Part model, mm, in its own coordinate system. Face numbers are marked on the shaded views. A direction names the side the tool comes from. Give positions to 0.01 mm unless a question says otherwise; leave off trailing zeros. Order: outer loops, then holes, each group sorted by start corner. A loop starts at its lowest first (then second) coordinate and runs counter-clockwise, first axis right, second up. Notation, with made-up numbers: (1.5, -8.5) - (31.5, -8.5) arc R17 cw to (31.5, 20.5) - close; hole circle Ø4 at (50, 31). An arc over 180 degrees is marked (long way). One line per item, written item: value.
```python
from build123d import *

# Parameters (mm, degrees)
SKETCH1_R           = 25
SKETCH1_R_2         = 22.5
BOSS_EXTRUDE1_DEPTH = 9.4
SKETCH2_R           = 25
BOSS_EXTRUDE2_DEPTH = 40
SKETCH3_W           = 55.38055132
SKETCH3_H           = 33.998264421
CUT_EXTRUDE1_DEPTH  = 36
SKETCH4_R           = 3.5
CUT_EXTRUDE2_DEPTH  = 36
CUT_EXTRUDE3_START  = -2
SKETCH5_R           = 3.5
SKETCH5_R_2         = 2.05
SKETCH5_R_3         = 1.95
CUT_EXTRUDE3_DEPTH  = 2
SKETCH5_3_R         = 1.95
CUT_EXTRUDE4_DEPTH  = 2
SKETCH6_W           = 12.45
SKETCH6_H           = 22.55
CUT_EXTRUDE5_DEPTH  = 42
SKETCH6_4_W         = 12.45
SKETCH6_4_H         = 4.85
CUT_EXTRUDE6_DEPTH  = 2.5
SKETCH6_5_W         = 12.45
SKETCH6_5_H         = 2.312362619
CUT_EXTRUDE7_DEPTH  = 28.5
SKETCH7_W           = 47.88210926
SKETCH7_H           = 3
BOSS_EXTRUDE3_DEPTH = 3
SKETCH8_W           = 47.88210926
SKETCH8_H           = 3
BOSS_EXTRUDE4_DEPTH = 4.7
FILLET1_R           = 5
FILLET2_R           = 2
FILLET3_R           = 2
BOSS_EXTRUDE5_DEPTH = 35
FILLET4_R           = 12
SKETCH10_R          = 1.8
CUT_EXTRUDE8_DEPTH  = 36


with BuildPart() as part:
    # Sketch1 → Boss-Extrude1 (new body)
    with BuildSketch(Plane(origin=(0, 0, 0), x_dir=(1, 0, 0), z_dir=(0, 1, 0))):
        with Locations(Location((0, 0, 0), (0, 0, 270))):
            Circle(SKETCH1_R)
        with Locations(Location((0, 0, 0), (0, 0, 270))):
            Circle(SKETCH1_R_2, mode=Mode.SUBTRACT)
    extrude(amount=BOSS_EXTRUDE1_DEPTH)

    # Sketch2 → Boss-Extrude2 (add)
    with BuildSketch(Plane(origin=(0, 9.4, 0), x_dir=(1, 0, 0), z_dir=(0, 1, 0))):
        with Locations(Location((0, 0, 0), (0, 0, 270))):
            Circle(SKETCH2_R)
    extrude(amount=BOSS_EXTRUDE2_DEPTH)

    # Sketch3 → Cut-Extrude1 (cut)
    with BuildSketch(Plane(origin=(0, 49.4, 0), x_dir=(1, 0, 0), z_dir=(0, 1, 0))):
        with Locations((-2.69027566, -9.800111221)):
            Rectangle(SKETCH3_W, SKETCH3_H)
    extrude(amount=-CUT_EXTRUDE1_DEPTH, mode=Mode.SUBTRACT)

    # Sketch4 → Cut-Extrude2 (cut)
    with BuildSketch(Plane.XZ.offset(-9.4)):
        with Locations(Location((0, 0, 0), (0, 0, 270))):
            Circle(SKETCH4_R)
    extrude(amount=-CUT_EXTRUDE2_DEPTH, mode=Mode.SUBTRACT)

    # Sketch5 → Cut-Extrude3 (cut)
    # profile 1 of 6: a face of its own
    with BuildSketch(Plane(origin=(0, 13.4, 0), x_dir=(1, 0, 0), z_dir=(0, 1, 0)).offset(CUT_EXTRUDE3_START)):
        with BuildLine():
            Line((-1.95, 6.45), (-14.05, 2.05))
            ThreePointArc((-14.05, 2.05), (-12.600431099, 1.449568901), (-12, 0))
            ThreePointArc((-12, 0), (-12.600431099, -1.449568901), (-14.05, -2.05))
            Line((-14.05, -2.05), (-1.95, -6.45))
            ThreePointArc((-1.95, -6.45), (0, -4.5), (1.95, -6.45))
            Line((1.95, -6.45), (16.45, -2.05))
            ThreePointArc((16.45, -2.05), (14.4, 0), (16.45, 2.05))
            Line((16.45, 2.05), (1.95, 6.45))
            ThreePointArc((1.95, 6.45), (0, 4.5), (-1.95, 6.45))
        make_face()
        with Locations(Location((0, 0, 0), (0, 0, 90))):
            Circle(SKETCH5_R, mode=Mode.SUBTRACT)
    # profile 2 of 6: a face of its own
    with BuildSketch(Plane(origin=(0, 13.4, 0), x_dir=(1, 0, 0), z_dir=(0, 1, 0)).offset(CUT_EXTRUDE3_START)):
        with BuildLine():
            ThreePointArc((-1.800407609, 7.199020989), (-1.912236235, 6.831906509), (-1.95, 6.45))
            ThreePointArc((-1.95, 6.45), (0, 4.5), (1.95, 6.45))
            ThreePointArc((1.95, 6.45), (1.912236235, 6.831906509), (1.800407609, 7.199020989))
            Line((1.800407609, 7.199020989), (-1.800407609, 7.199020989))
        make_face()
    # profile 3 of 6: a face of its own
    with BuildSketch(Plane(origin=(0, 13.4, 0), x_dir=(1, 0, 0), z_dir=(0, 1, 0)).offset(CUT_EXTRUDE3_START)):
        with BuildLine():
            ThreePointArc((1.800407609, 7.199020989), (0, 8.4), (-1.800407609, 7.199020989))
            Line((-1.800407609, 7.199020989), (1.800407609, 7.199020989))
        make_face()
    # profile 4 of 6: a face of its own
    with BuildSketch(Plane(origin=(0, 13.4, 0), x_dir=(1, 0, 0), z_dir=(0, 1, 0)).offset(CUT_EXTRUDE3_START)):
        with Locations((-14.05, 0)):
            Circle(SKETCH5_R_2)
    # profile 5 of 6: a face of its own
    with BuildSketch(Plane(origin=(0, 13.4, 0), x_dir=(1, 0, 0), z_dir=(0, 1, 0)).offset(CUT_EXTRUDE3_START)):
        with Locations((16.45, 0)):
            Circle(SKETCH5_R_2)
    # profile 6 of 6: a face of its own
    with BuildSketch(Plane(origin=(0, 13.4, 0), x_dir=(1, 0, 0), z_dir=(0, 1, 0)).offset(CUT_EXTRUDE3_START)):
        with Locations((0, -6.45)):
            Circle(SKETCH5_R_3)
    extrude(amount=CUT_EXTRUDE3_DEPTH, mode=Mode.SUBTRACT)

    # Sketch5<3> → Cut-Extrude4 (cut)
    with BuildSketch(Plane(origin=(0, 13.4, 0), x_dir=(1, 0, 0), z_dir=(0, 1, 0))):
        with Locations((0, 6.45)):
            Circle(SKETCH5_3_R)
    extrude(amount=CUT_EXTRUDE4_DEPTH, mode=Mode.SUBTRACT)

    # Sketch6 → Cut-Extrude5 (cut)
    with BuildSketch(Plane.XY.offset(-7.199020989)):
        with Locations((0, 35.812637381)):
            Rectangle(SKETCH6_W, SKETCH6_H)
    extrude(amount=-CUT_EXTRUDE5_DEPTH, mode=Mode.SUBTRACT)

    # Sketch6<4> → Cut-Extrude6 (cut)
    with BuildSketch(Plane.XY.offset(-7.199020989)):
        with Locations((0, 22.112637381)):
            Rectangle(SKETCH6_4_W, SKETCH6_4_H)
    extrude(amount=-CUT_EXTRUDE6_DEPTH, mode=Mode.SUBTRACT)

    # Sketch6<5> → Cut-Extrude7 (cut)
    with BuildSketch(Plane.XY.offset(-7.199020989)):
        with Locations((0, 48.243818691)):
            Rectangle(SKETCH6_5_W, SKETCH6_5_H)
    extrude(amount=-CUT_EXTRUDE7_DEPTH, mode=Mode.SUBTRACT)

    # Sketch7 → Boss-Extrude3 (add)
    with BuildSketch(Plane.XY.offset(-7.199020989)):
        with Locations((0, 18.187637381)):
            Rectangle(SKETCH7_W, SKETCH7_H)
    extrude(amount=BOSS_EXTRUDE3_DEPTH)

    # Sketch8 → Boss-Extrude4 (add)
    with BuildSketch(Plane(origin=(0, 19.687637381, 0), x_dir=(1, 0, 0), z_dir=(0, 1, 0))):
        with Locations((0, 5.699020989)):
            Rectangle(SKETCH8_W, SKETCH8_H)
    extrude(amount=BOSS_EXTRUDE4_DEPTH)

    # Fillet1
    fillet1_edges = [part.edges().sort_by_distance(p)[0] for p in [
        (-15.083027315, 49.4, -7.199020989),
        (15.083027315, 49.4, -7.199020989),
    ]]
    fillet(fillet1_edges, radius=FILLET1_R)

    # Fillet2
    fillet2_edges = [part.edges().sort_by_distance(p)[0] for p in [
        (6.225, 36.96881869, -24.212587119),
        (-6.225, 36.96881869, -24.212587119),
    ]]
    fillet(fillet2_edges, radius=FILLET2_R)

    # Fillet3
    fillet3_edges = [part.edges().sort_by_distance(p)[0] for p in [
        (-23.94105463, 20.537637381, -4.199020989),
        (0, 16.687637381, -4.199020989),
        (23.94105463, 20.537637381, -4.199020989),
    ]]
    fillet(fillet3_edges, radius=FILLET3_R)

    # Sketch9 → Boss-Extrude5 (add)
    with BuildSketch(Plane(origin=(0, 13.4, 0), x_dir=(1, 0, 0), z_dir=(0, 1, 0))):
        with BuildLine():
            Line((18.619699915, -16.682529037), (-18.619699915, -16.682529037))
            ThreePointArc((-18.619699915, -16.682529037), (0, -25), (18.619699915, -16.682529037))
        make_face()
    extrude(amount=BOSS_EXTRUDE5_DEPTH)

    # Fillet4
    # the kernel refuses this fillet: 12 mm, written as the material it takes off along each edge
    with BuildSketch(Plane(origin=(0, 48.4, 0), x_dir=(-0.8915807568580754, 0, -0.4528617382826481), z_dir=(0.4528617382826481, 0, -0.8915807568580754))) as fillet4_piece_1_section:
        with BuildLine():
            CenterArc((25 - FILLET4_R, -FILLET4_R), FILLET4_R, 0, 90)
            Line((25 - FILLET4_R, 0), (25, 0))
            Line((25, 0), (25, -FILLET4_R))
        make_face()
    fillet4_piece_1 = revolve(axis=Axis((0, 48.4, 0), (0, 1, 0)), revolution_arc=233.854877773, mode=Mode.PRIVATE)
    fillet4_piece_1 = split(fillet4_piece_1, bisect_by=Plane(origin=(0, 43.523140853, 16.682529037), z_dir=(0, 0, 1)), keep=Keep.TOP, mode=Mode.PRIVATE)
    add(fillet4_piece_1, mode=Mode.SUBTRACT)

    # Sketch10 → Cut-Extrude8 (cut)
    with BuildSketch(Plane(origin=(0, 0, 16.682529037), x_dir=(-1, 0, 0), z_dir=(0, 0, -1))):
        with Locations((0, 40.29)):
            Circle(SKETCH10_R)
    extrude(amount=-CUT_EXTRUDE8_DEPTH, mode=Mode.SUBTRACT)


solid = part.part
```
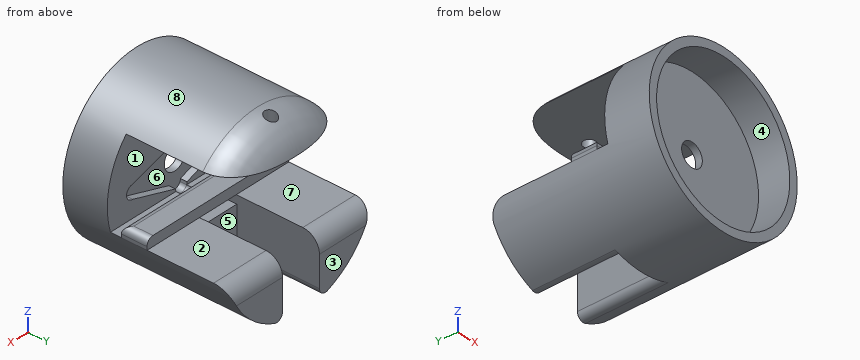
1) Slice it at D-D on y = 40.29. Write the cut outline in (x, z) (3 decimals).
Answer:
outline: (-23.941, -7.199) arc R25 ccw to (-8.94, -23.347) arc R2 ccw to (-6.225, -21.479) - (-6.225, -7.199) - close; (-17.74, 16.683) - (-1.8, 16.683) - (-1.8, 24.285) arc R24.352 ccw to start; (1.8, 16.683) - (17.74, 16.683) arc R24.352 ccw to (1.8, 24.285) - close; (6.225, -21.479) arc R2 ccw to (8.94, -23.347) arc R25 ccw to (23.941, -7.199) - (6.225, -7.199) - close
2) Drop flat-ended pins along their axis: P1, Ø12, axis at x = -17.5, y = 20, coming from the -Z side; P2, Ø6.5, axis at x = -8, y = 20.5, coming from the +Z side; P3, Ø4, axis at x = 16, y = 30.5, coming from the -Z side; P4, Ø1, axis at y = 43, z = 14.5, coming from the +X side. Give the stop position or say it passes through.
Answer:
P1: stops at z = -22.2
P2: stops at z = 24.54
P3: stops at z = -20.71
P4: passes through
3) Slice it at B-B on z = 0. Write the cut outline in (x, y), then the cut area to 3 significant figures.
Answer:
outline: (-25, 0) - (-22.5, 0) - (-22.5, 9.4) - (-3.5, 9.4) - (-3.5, 11.4) - (-16.1, 11.4) - (-16.1, 13.4) - (-25, 13.4) - close; (3.5, 9.4) - (22.5, 9.4) - (22.5, 0) - (25, 0) - (25, 13.4) - (18.5, 13.4) - (18.5, 11.4) - (3.5, 11.4) - close
area: 164 mm2
4) Slice it at C-C on x = 0. Count the separate pieces of the cut face and the enclosed holes in it, then the cut area to 3 significant figures.
Answer:
separate pieces: 3
enclosed holes: 0
area: 639 mm2
5) Two-plate mould, pull along X, no slides. Class the marked faces 6, 7 and 8: pulls with the +X half, pulls with the -X half, needs draft (parallel to the pull), parting line crosses it, or undercut.
Answer:
face 6: undercut
face 7: needs draft
face 8: parting line crosses it
6) Slice it at A-A on y = 21.5. Write the cut outline in (x, z) (3 decimals), then the cut area to 3 significant figures.
Answer:
outline: (-23.941, -7.199) arc R25 ccw to (23.941, -7.199) - (23.941, -6.199) arc R2 ccw to (21.941, -4.199) - (-21.941, -4.199) arc R2 ccw to (-23.941, -6.199) - close; (-18.62, 16.683) - (18.62, 16.683) arc R25 ccw to start; hole (-6.225, -9.699) - (6.225, -9.699) - (6.225, -7.199) - (-6.225, -7.199) - close
area: 952 mm2
7) Wall check: line 1 along Z through (x, y) = (0, 10.7); line 2 along X through (y, z) = (3, 0); line 3 along Z through (x, y) = (0, 24.5). Give the ranges that are in metal, low to high. Write a range as [from, to].
Answer:
line 1: z = [-25, -3.5], [3.5, 25]
line 2: x = [-25, -22.5], [22.5, 25]
line 3: z = [-25, -9.7], [16.68, 25]
8) Which spindle directions (+Z, -Z, +X, -X, +Y, -Y) get a long thin tool onto all of the face, cutting with end or side? Do the marked faces 1, 2, 3, 4 and 5. Say none if no direction does.
Answer:
face 1: +X, -X
face 2: +X, -X, +Y
face 3: +Z, -Z, +X, -X, +Y
face 4: -Y
face 5: -Z, +Y
